Check sheet for the drawn part. Datum: minimum x, y, z corner. Units: mm. A direction names the side the tool comes from. Round coordinates to 2 decimals unless told otherwise and drop trailing zeros. Order: outer loops, then holes, each group sorted by start corner. A loop starts at its lowest first (then second) coordinate and runs counter-clockwise, first axis right, second up.
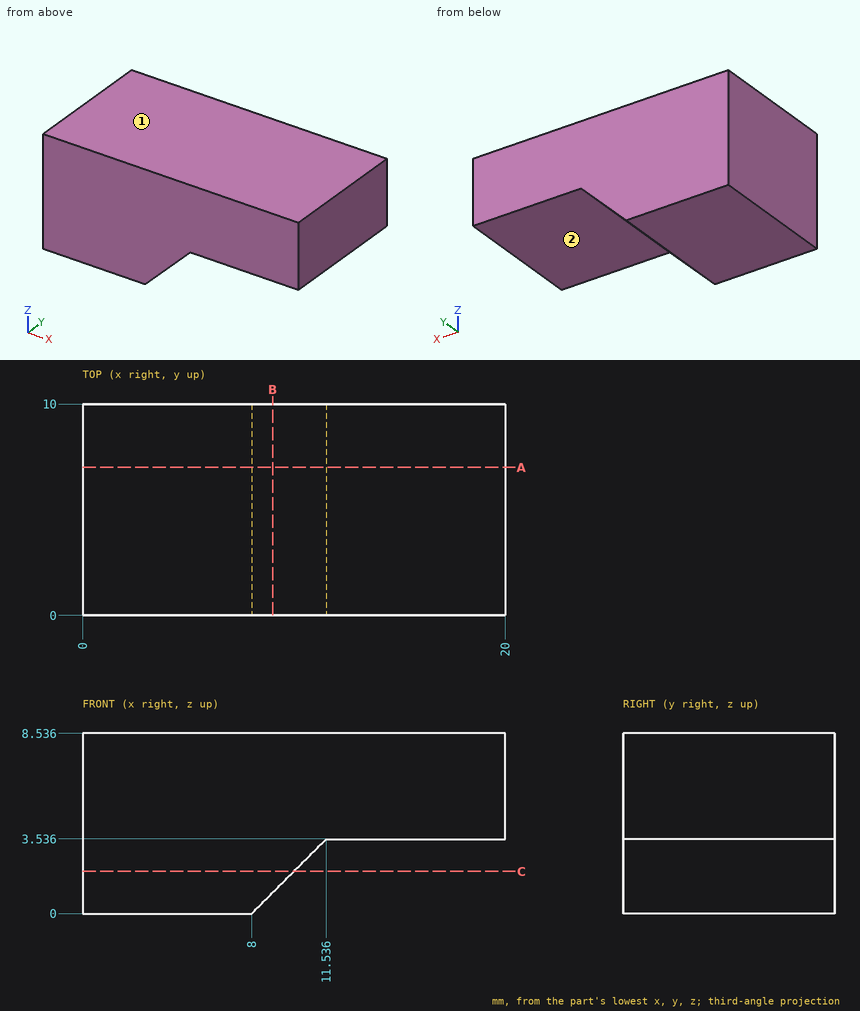
(1) Material ranges on line 1 (Z direction, x = 17.25, y = 4.75) (1 decimal); line 2 (X direction, y = 2.75, z = 2); line 3 (X direction, y = 5.25, z = 1.75), recorded low to high.
Returned:
line 1: z = 3.5 to 8.5
line 2: x = 0 to 10
line 3: x = 0 to 9.75
(2) Sectioned sample at C-C, the plane z = 2. Record the cut outline in (x, y), and give its area (3 significant figures).
Returned:
outline: (0, 0) - (10, 0) - (10, 10) - (0, 10) - close
area: 100 mm2
(3) Sectioned sample at A-A, the plane y = 7. Record the cut outline in (x, z) (1 decimal).
Returned:
outline: (0, 0) - (8, 0) - (11.5, 3.5) - (20, 3.5) - (20, 8.5) - (0, 8.5) - close
(4) Sectioned sample at B-B, the plane x = 9. Record the cut outline in (y, z) (1 decimal).
Returned:
outline: (0, 1) - (10, 1) - (10, 8.5) - (0, 8.5) - close
(5) Set-up check for the marked faces 1 and 2: record each of +Z, -Z, +X, -X, +Y, -Y from which the full face is reachable in a straight line by a thin tool's end or side.
Returned:
face 1: +Z, +X, -X, +Y, -Y
face 2: -Z, +X, +Y, -Y
